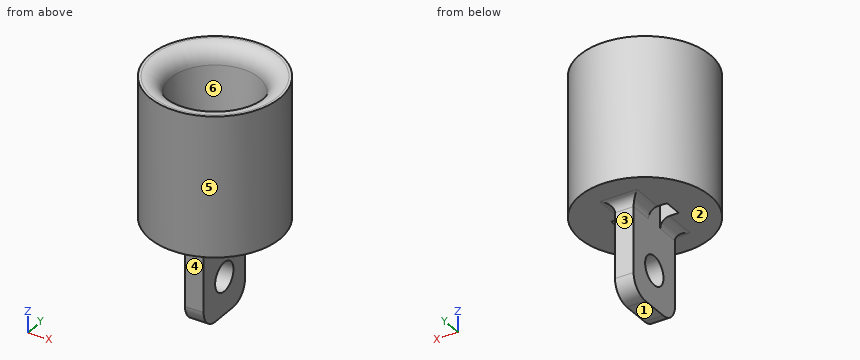
```python
from build123d import *

# Parameters (mm, degrees)
SKETCH001_W     = 2
SKETCH001_H     = 7
PAD_DEPTH       = 10
FILLET_R        = 1
FILLET001_R     = 1
FILLET002_R     = 1
FILLET003_R     = 1
FILLET004_R     = 2
SKETCH002_R     = 1.55
POCKET_DEPTH    = 5
SKETCH003_W     = 2
SKETCH003_H     = 2
POCKET001_DEPTH = 2.5


with BuildPart() as part:
    # Sketch → Revolution (revolve)
    with BuildSketch(Plane.XZ):
        Polygon((0, 0), (0, 2), (3, 2), (5, 15), (7, 15), (7, 0), align=None)
    revolve(axis=Axis((0, 0, 0), (0, 0, 1)))

    # Sketch001 (on Face5 of Revolution) → Pad (new body)
    with BuildSketch(Plane(origin=(0, 0, 0), x_dir=(1, 0, 0), z_dir=(0, 0, -1))):
        Rectangle(SKETCH001_W, SKETCH001_H)
    extrude(amount=PAD_DEPTH)

    # Fillet
    fillet_edges = [part.edges().sort_by_distance(p)[0] for p in [
        (1, 0, 0),
    ]]
    fillet(fillet_edges, radius=FILLET_R)

    # Fillet001
    fillet001_edges = [part.edges().sort_by_distance(p)[0] for p in [
        (-1, 0, 0),
    ]]
    fillet(fillet001_edges, radius=FILLET001_R)

    # Fillet002
    fillet002_edges = [part.edges().sort_by_distance(p)[0] for p in [
        (0, -3.5, 0),
    ]]
    fillet(fillet002_edges, radius=FILLET002_R)

    # Fillet003
    fillet003_edges = [part.edges().sort_by_distance(p)[0] for p in [
        (0, 3.5, 0),
    ]]
    fillet(fillet003_edges, radius=FILLET003_R)

    # Fillet004
    fillet004_edges = [part.edges().sort_by_distance(p)[0] for p in [
        (-5, 0, 15),
        (0, 3.5, -10),
        (0, -3.5, -10),
    ]]
    fillet(fillet004_edges, radius=FILLET004_R)

    # Sketch002 → Pocket (cut)
    with BuildSketch(Plane(origin=(-1, 0, 0), x_dir=(0, 0, -1), z_dir=(-1, 0, 0))):
        with Locations((6, 0)):
            Circle(SKETCH002_R)
    extrude(amount=-POCKET_DEPTH, mode=Mode.SUBTRACT)

    # Sketch003 (on Face12 of Pocket) → Pocket001 (cut, symmetric)
    with BuildSketch(Plane(origin=(0, 0, 0), x_dir=(1, 0, 0), z_dir=(0, 0, -1))):
        with Locations((-2, 0)):
            Rectangle(SKETCH003_W, SKETCH003_H)
        with Locations((2, 0)):
            Rectangle(SKETCH003_W, SKETCH003_H)
    extrude(amount=POCKET001_DEPTH, both=True, mode=Mode.SUBTRACT)


solid = part.part
```
Work out the finished part from the listing and answer in its coordinate system (mm). Face numbers are marked on the shaded views. A direction names the side the tool comes from. Give positions to 0.01 mm unless a question says otherwise; leave off trailing zeros. Loops run counter-clockwise (first coordinate to the right, second up) from the corner with the lowest first, then second, coordinate; pieces in that order, holes last. Notation, with made-up numbers: (88.5, 0) -> (102.5, 0) arc R14 cw to (102.5, 20) -> close; hole circle Ø10 at (72, -14). An arc over 180 degrees is marked (long way). Put each result on its own line as item: value. Start each with the question number.
Item 1: The part is cut by section A-A (z = -6). Give the vertices of the cut face in (x, y), then the cut area to 3 significant figures.
Item 2: The part is cut by section D-D (z = 1). Give the vertices of the cut face in (x, y), then the cut area to 3 significant figures.
Item 3: Which of the six approach directions +Z, -Z, +X, -X, +Y, -Y give full straight-line access (tool end or side, diameter ignored) to the marked faces 1, 2 and 3?
Item 4: Find the intervals of material crossed by L1, parallel to Z at x = 0.35, y = 0; L2, parallel to Y at x = -0.4, z = -6; L3, parallel to X at y = 0.5, z = 1.5, in increasing order. Write a range as [from, to].
Item 5: The mould has two halves that part along X. Classify the marked faces 4, 5 and 6: released by +X, released by -X, zero draft, split by the parting line, or undercut.
Item 6: Each of these flat-tipped pins is pushed along its axis until it touches: P1, Ø1, axis at x = 0, z = -4.5, coming from the +Y side; P2, Ø2, axis at x = -3, y = 3, coming from the +Z side; P3, Ø1.5, axis at y = 1.5, z = -4.5, coming from the +X side; P4, Ø4, axis at x = 2, y = 5, coming from the +Z side. Where does it stop, or does it pass through?
Item 7: The part is cut by section B-B (y = 0). Give the vertices of the cut face in (x, z).
Item 8: The part is cut by section C-C (x = 0). Give the vertices of the cut face in (y, z).
Answers below:
1. outline: (-1, -3.5) -> (1, -3.5) -> (1, -1.55) -> (-1, -1.55) -> close; (-1, 1.55) -> (1, 1.55) -> (1, 3.5) -> (-1, 3.5) -> close
1. area: 7.80 mm2
2. outline: circle Ø14 at (0, 0); hole (-3, -1) -> (-1, -1) -> (-1, 1) -> (-3, 1) -> close; hole (1, -1) -> (3, -1) -> (3, 1) -> (1, 1) -> close
2. area: 146 mm2
3. face 1: -Z, +X, -X, +Y, -Y
3. face 2: -Z
3. face 3: -Z, +X, -X, +Y
4. L1: [-10, -7.55], [-4.45, 2]
4. L2: [-3.5, -1.55], [1.55, 3.5]
4. L3: [-6.98, -3], [-1, 1], [3, 6.98]
5. face 4: zero draft
5. face 5: split by the parting line
5. face 6: undercut
6. P1: y = 3.5
6. P2: z = 14.35
6. P3: x = 1
6. P4: z = 15
7. outline: (-7, 0) -> (-3, 0) -> (-3, 2) -> (-4.74, 13.3) arc R2 ccw to (-6.72, 15) -> (-7, 15) -> close; (-1, -10) -> (1, -10) -> (1, -7.55) -> (-1, -7.55) -> close; (-1, -4.45) -> (1, -4.45) -> (1, 2) -> (-1, 2) -> close; (3, 0) -> (7, 0) -> (7, 15) -> (6.72, 15) arc R2 ccw to (4.74, 13.3) -> (3, 2) -> close
8. outline: (-7, 0) -> (-4.5, 0) arc R1 cw to (-3.5, -1) -> (-3.5, -8) arc R2 ccw to (-1.5, -10) -> (1.5, -10) arc R2 ccw to (3.5, -8) -> (3.5, -1) arc R1 cw to (4.5, 0) -> (7, 0) -> (7, 15) -> (6.72, 15) arc R2 ccw to (4.74, 13.3) -> (3, 2) -> (-3, 2) -> (-4.74, 13.3) arc R2 ccw to (-6.72, 15) -> (-7, 15) -> close; hole circle Ø3.1 at (0, -6)
